Autodesk Inventor part; units mm, degrees
ref_plane "YZ Plane" through (0, 0, 0) normal (1, 0, 0) x (0, 1, 0)
ref_plane "XZ Plane" through (0, 0, 0) normal (0, 1, 0) x (-1, 0, 0)
ref_plane "XY Plane" through (0, 0, 0) normal (0, 0, 1) x (1, 0, 0)
sketch "Sketch4" plane through (0, 0, 0) normal (0, 1, 0) x (-1, 0, 0)
  line L0 (47, 47) -> (-47, 47)
  line L1 (-47, 47) -> (-47, -47)
  line L2 (-47, -47) -> (47, -47)
  line L3 (47, -47) -> (47, 47)
  line L4 (47, 47) -> (-47, -47) construction
  line L5 (-47, 47) -> (47, -47) construction
  point P0 (0, 0)
  dimension "d52" = 94
  dimension "d53" = 94
extrude "Extrusion5" add sketch "Sketch4" along normal blind 2
sketch "Sketch6" plane through (0, 0, 0) normal (0, -1, 0) x (1, 0, 0)
  line L0 (-46.5, -40) -> (-45.5, -40)
  line L1 (-45.5, -40) -> (-45.5, -20)
  line L2 (-45.5, -20) -> (-46.5, -20)
  line L3 (-46.5, -20) -> (-46.5, -40)
  line L4 (-45.5, 20) -> (-46.5, 20)
  line L5 (-46.5, 20) -> (-46.5, 40)
  line L6 (-46.5, 40) -> (-45.5, 40)
  line L7 (-45.5, 40) -> (-45.5, 20)
  line L8 (-40, 46.5) -> (-20, 46.5)
  line L9 (-20, 46.5) -> (-20, 45.5)
  line L10 (-20, 45.5) -> (-40, 45.5)
  line L11 (-40, 45.5) -> (-40, 46.5)
  line L12 (40, 46.5) -> (20, 46.5)
  line L13 (20, 46.5) -> (20, 45.5)
  line L14 (20, 45.5) -> (40, 45.5)
  line L15 (40, 45.5) -> (40, 46.5)
  line L16 (45.5, 40) -> (46.5, 40)
  line L17 (46.5, 40) -> (46.5, 20)
  line L18 (46.5, 20) -> (45.5, 20)
  line L19 (45.5, 20) -> (45.5, 40)
  line L20 (45.5, -40) -> (46.5, -40)
  line L21 (46.5, -40) -> (46.5, -20)
  line L22 (46.5, -20) -> (45.5, -20)
  line L23 (45.5, -20) -> (45.5, -40)
  line L24 (40, -45.5) -> (20, -45.5)
  line L25 (20, -45.5) -> (20, -46.5)
  line L26 (20, -46.5) -> (40, -46.5)
  line L27 (40, -46.5) -> (40, -45.5)
  line L28 (-40, -45.5) -> (-20, -45.5)
  line L29 (-20, -45.5) -> (-20, -46.5)
  line L30 (-20, -46.5) -> (-40, -46.5)
  line L31 (-40, -46.5) -> (-40, -45.5)
  line L32 (-47, 47) -> (-47, -47)
  line L33 (47, 47) -> (-47, 47)
  line L34 (47, -47) -> (47, 47)
  line L35 (-47, -47) -> (47, -47)
  point P0 (0, 0)
  point P1 (-46, 40)
  point P2 (-46, 20)
  point P3 (46, 40)
  point P4 (46, -40)
  point P5 (-40, -46)
  point P6 (-46, -40)
  dimension "d123" = 1
  dimension "d124" = 20
  dimension "d119" = 1
  dimension "d118" = 20
  dimension "d116" = 20
  dimension "d117" = 1
  dimension "d112" = 20
  dimension "d113" = 1
  dimension "d108" = 1
  dimension "d109" = 20
  dimension "d104" = 1
  dimension "d105" = 20
  dimension "d101" = 20
  dimension "d102" = 1
  dimension "d97" = 20
  dimension "d98" = 1
  dimension "d114" = 7
  dimension "d115" = 0.5
  dimension "d111" = 0.5
  dimension "d110" = 7
  dimension "d107" = 7
  dimension "d106" = 0.5
  dimension "d103" = 0.5
  dimension "d95" = 7
  dimension "d99" = 7
  dimension "d100" = 0.5
  dimension "d96" = 0.5
  dimension "d94" = 7
  dimension "d93" = 7
  dimension "d122" = 0.5
  dimension "d120" = 7
  dimension "d121" = 0.5
extrude "Extrusion7" add sketch "Sketch6" along normal blind 1 contours L3 L2 L1 L0 | L4 L5 L6 L7 | L8 L9 L10 L11 | L15 L14 L13 L12 | L16 L17 L18 L19 | L23 L22 L21 L20 | L27 L26 L25 L24 | L28 L29 L30 L31
fillet "Fillet9" radius 1 1 edges at (47, 1, -47)
fillet "Fillet10" radius 1 1 edges at (-47, 1, -47)
fillet "Fillet11" radius 1 1 edges at (-47, 1, 47)
fillet "Fillet12" radius 1 1 edges at (47, 1, 47)
fillet "Fillet13" radius 1 8 edges at (-46.7071, 2, -46.7071) (-47, 2, 0) (-46.7071, 2, 46.7071) (0, 2, 47) (46.7071, 2, 46.7071) (47, 2, 0) (46.7071, 2, -46.7071) (0, 2, -47)
properties part number "block_main" material "PC/ABS Plastic"
Build history of the part. All positions in model axes, mm. Round coordinates to 2 decimals unless told otherwise and drop trailing zeros. Loops run counter-clockwise (first coordinate to the right, second up) from the corner with the lowest first, then second, coordinate; pieces in that order, holes last. Notation, with made-up numbers: M 8.5,66 L 48.5,66 A31 cw 48.5,101 Z; hole C 88.25,76.25 d1. An arc over 180 degrees is marked long. Answer as CSV lines item,"result".
1. Cut at B-B on z = 29. Write the cut outline in (x, y), then the cut area to 3 significant figures.
Resolved:
outline,"M -47,0 L -46.5,0 L -46.5,-1 L -45.5,-1 L -45.5,0 L 45.5,0 L 45.5,-1 L 46.5,-1 L 46.5,0 L 47,0 L 47,1 A1 ccw 46,2 L -46,2 A1 ccw -47,1 Z"
area,"190 mm²"
2. Flat gauge pins, fed straight in: P1, Ø0.5, axis at x = 30.5, y = -0.5, coming from the -Z side; P2, Ø0.8, axis at y = -0.5, z = -25.5, coming from the -X side; P3, Ø0.5, axis at y = -0.5, z = -46, coming from the +X side. Where does each tip first touch, or does it go through?
Resolved:
P1,"stops at z = -46.5"
P2,"stops at x = -46.5"
P3,"stops at x = 40"
3. Cut at A-A on x = 29.5. Write the cut outline in (y, z).
Resolved:
outline,"M -1,-46.5 L 0,-46.5 L 0,-47 L 1,-47 A1 ccw 2,-46 L 2,46 A1 ccw 1,47 L 0,47 L 0,46.5 L -1,46.5 L -1,45.5 L 0,45.5 L 0,-45.5 L -1,-45.5 Z"
4. Two-plate mould, pull along Z, no slides. Class faces 1 (the flat face through (1, 0, 1)), 2 (the flat face through (1, 2, 1)): released by +Z, released by -Z, zero draft, split by the parting line, or undercut.
Resolved:
face 1,"undercut"
face 2,"zero draft"
5. Cut at D-D on z = 2.5. Write the cut outline in (x, y), then the cut area to 3 significant figures.
Resolved:
outline,"M -47,0 L 47,0 L 47,1 A1 ccw 46,2 L -46,2 A1 ccw -47,1 Z"
area,"188 mm²"
6. Cut at C-C on x = -15. Write the cut outline in (y, z).
Resolved:
outline,"M 0,-47 L 1,-47 A1 ccw 2,-46 L 2,46 A1 ccw 1,47 L 0,47 Z"
7. Wall check: probe 1 along Z at (x, y) = (-26, -0.1); probe 2 along Y at (x, z) = (-5, -25.5). Give the ranges that are in metal, low to high. Write a range as [from, to].
Resolved:
probe 1,"z = [-46.5, -45.5], [45.5, 46.5]"
probe 2,"y = [0, 2]"
